Part model, mm, in its own coordinate system. Face numbers are marked on the shaded views. A direction names the side the tool comes from. Round coordinates to 2 decimals unless told otherwise and drop trailing zeros. Order: outer loops, then holes, each group sorted by start corner. A loop starts at its lowest first (then second) coordinate and runs counter-clockwise, first axis right, second up. Notation, with made-up numbers: (28.25, -5.75) - (41.25, -5.75) arc R23 ccw to (41.25, 18.25) - close; hole circle Ø3 at (-37, 78). An arc over 180 degrees is marked (long way). Answer as a JSON object with one key per item and string values.
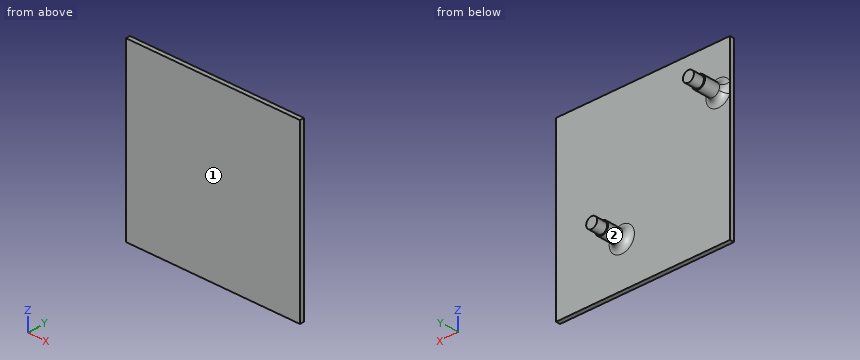
```python
from build123d import *

# Parameters (mm, degrees)
SKETCH1_W           = 55
SKETCH1_H           = 55
BOSS_EXTRUDE1_DEPTH = 2
SKETCH2_R           = 3
BOSS_EXTRUDE2_DEPTH = 10
FILLET1_R           = 2.8
SKETCH3_R           = 2.5
BOSS_EXTRUDE3_DEPTH = 5


with BuildPart() as part:
    # Sketch1 → Boss-Extrude1 (new body)
    with BuildSketch(Plane(origin=(0, 0, 0), x_dir=(1, 0, 0), z_dir=(0, 1, 0))):
        Polygon((52.5, 40), (52.5, -40), (-27.5, -40), (-27.5, -27.5), (27.5, -27.5), (27.5, 27.5), (-27.5, 27.5), (-27.5, 40), align=None)
        Rectangle(SKETCH1_W, SKETCH1_H)
    extrude(amount=BOSS_EXTRUDE1_DEPTH)

    # Sketch2 → Boss-Extrude2 (add)
    with BuildSketch(Plane(origin=(0, 2, 0), x_dir=(1, 0, 0), z_dir=(0, 1, 0))):
        with Locations(Location((-22.25, -19.75, 0), (0, 0, 270))):
            Circle(SKETCH2_R)
        with Locations(Location((22.25, 19.75, 0), (0, 0, 270))):
            Circle(SKETCH2_R)
    extrude(amount=BOSS_EXTRUDE2_DEPTH)

    # Fillet1
    fillet1_edges = [part.edges().sort_by_distance(p)[0] for p in [
        (-22.25, 2, 16.75),
        (22.25, 2, -22.75),
    ]]
    fillet(fillet1_edges, radius=FILLET1_R)

    # Sketch3 → Boss-Extrude3 (add)
    with BuildSketch(Plane(origin=(0, 12, 0), x_dir=(1, 0, 0), z_dir=(0, 1, 0))):
        with Locations(Location((-22.25, -19.75, 0), (0, 0, 270))):
            Circle(SKETCH3_R)
        with Locations(Location((22.25, 19.75, 0), (0, 0, 270))):
            Circle(SKETCH3_R)
    extrude(amount=BOSS_EXTRUDE3_DEPTH)


solid = part.part
```
Item 1: Cut at B-B (y = 6.5). Write the cut outline in (x, z), plus the area to 3 significant figures.
Taken from the geometry:
{"outline": "circle Ø6 at (-22.25, 19.75); circle Ø6 at (22.25, -19.75)", "area": "56.5 mm2"}
Item 2: Cut at A-A (x = -22.25). Write the cut outline in (y, z), plus the area to 3 significant figures.
Taken from the geometry:
{"outline": "(0, -40) - (2, -40) - (2, 13.95) arc R2.8 cw to (4.8, 16.75) - (12, 16.75) - (12, 17.25) - (17, 17.25) - (17, 22.25) - (12, 22.25) - (12, 22.75) - (4.8, 22.75) arc R2.8 cw to (2, 25.55) - (2, 40) - (0, 40) - close", "area": "248 mm2"}
Item 3: Probe L1, parallel to Y at x = 36, z = 5; L2, parallel to X at y = 9, z = 21.5; L3, parallel to X at y = 6, z = 18.5. List the from-to ranges inside material, lowest first. Write a range as from..to.
Taken from the geometry:
{"L1": "0..2", "L2": "-24.69..-19.81", "L3": "-24.98..-19.52"}
Item 4: Cut at D-D (y = 13.5). Write the cut outline in (x, z).
Taken from the geometry:
{"outline": "circle Ø5 at (-22.25, 19.75); circle Ø5 at (22.25, -19.75)"}
Item 5: Tool access for the marked faces 1 and 2: list every direction of +Z, -Z, +X, -X, +Y, -Y with a clear straight run to the whole face (end or side of a thin tool).
Taken from the geometry:
{"face 1": "+Z, -Z, +X, -X, -Y", "face 2": "+Y"}
Item 6: Cut at C-C (z = -19.75). Write the cut outline in (x, y).
Taken from the geometry:
{"outline": "(-27.5, 0) - (52.5, 0) - (52.5, 2) - (28.05, 2) arc R2.8 cw to (25.25, 4.8) - (25.25, 12) - (24.75, 12) - (24.75, 17) - (19.75, 17) - (19.75, 12) - (19.25, 12) - (19.25, 4.8) arc R2.8 cw to (16.45, 2) - (-27.5, 2) - close"}
Item 7: Drop flat-ended pins along their axis: P1, Ø10, axis at x = 23, y = 14.5, coming from the +Z side; P2, Ø10, axis at y = 9.5, z = 16, coming from the -X side; P3, Ø2, axis at x = 11.5, z = -15, coming from the +Y side. Give the stop position or say it passes through.
Taken from the geometry:
{"P1": "z = -16.75", "P2": "x = -25.25", "P3": "y = 2"}
